Job drawing, mm, ordinate dimensions from the low corner. One solid piece. Round coordinates to 2 decimals unless told otherwise and drop trailing zeros. Write each loop counter-clockwise with the first axis right and the second up, starting at its lowest first coordinate (ties: lowest second). Pieces come first, ordered by that corner, then holes. Notation, with made-up numbers: (-21, -12.75) - (22, -12.75) arc R31 ccw to (22, 26.25) - close; hole circle Ø6 at (46, -2.75). An arc over 180 degrees is marked (long way). Write each question's results on one line, items separated by ' | '.
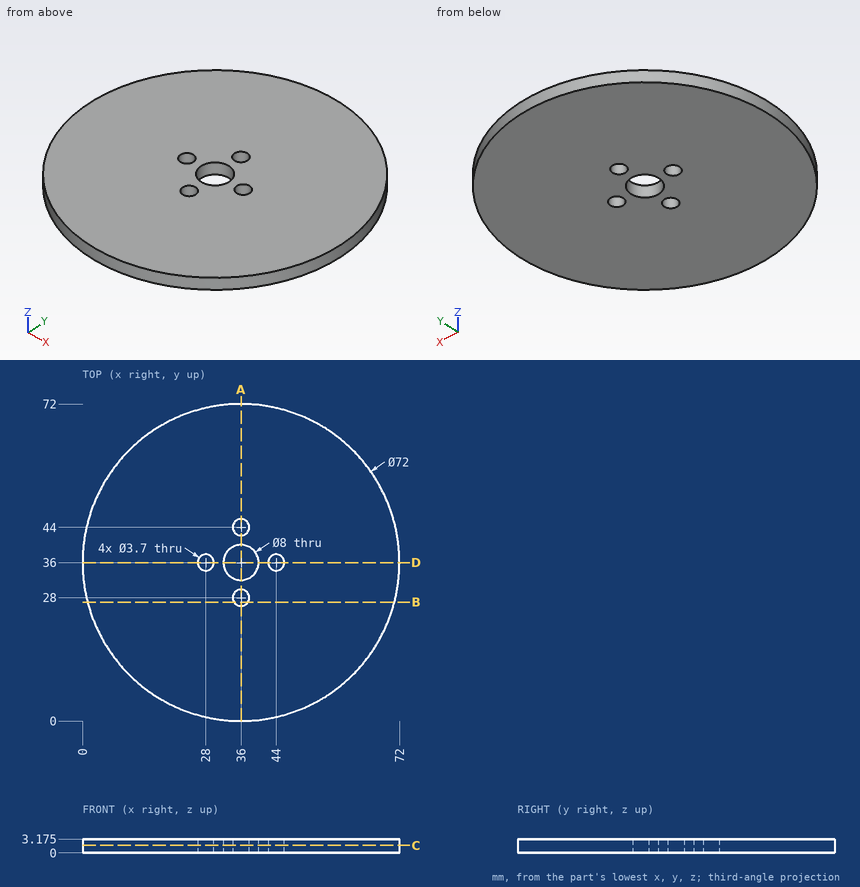
(1) Slice it at C-C, the plane z = 1.7. Write the cut outline in (x, y).
Worked answers:
outline: circle Ø72 at (36, 36); hole circle Ø3.7 at (28, 36); hole circle Ø8 at (36, 36); hole circle Ø3.7 at (36, 28); hole circle Ø3.7 at (36, 44); hole circle Ø3.7 at (44, 36)
(2) Flat gauge pins, fed straight in: pin 1 Ø10.5 at (x, y) = (36, 36) entering from +Z (3 decimals); pin 2 Ø3.5 at (x, y) = (36, 28) entering from -Z; pin 3 Ø1.5 at (y, z) = (41, 2.5) entering from -X. Where does each tip first touch, or does it go through?
Worked answers:
pin 1: stops at z = 3.175 | pin 2: passes through | pin 3: stops at x = 0.25
(3) Drill centre lines: probe 1 along Y at (x, z) = (36, 0.9); probe 2 along Y at (x, z) = (28, 1.9); probe 3 along X at (y, z) = (27.5, 2.05). Where is each one in solid material? Low to high. Write a range as [from, to].
Worked answers:
probe 1: y = [0, 26.15], [29.85, 32], [40, 42.15], [45.85, 72] | probe 2: y = [0.9, 34.15], [37.85, 71.1] | probe 3: x = [1.02, 34.22], [37.78, 70.98]
(4) Slice it at B-B, the plane y = 27. Write the cut outline in (x, z) (3 decimals), and give its area (3 significant figures).
Worked answers:
outline: (1.143, 0) - (34.444, 0) - (34.444, 3.175) - (1.143, 3.175) - close; (37.556, 0) - (70.857, 0) - (70.857, 3.175) - (37.556, 3.175) - close | area: 211 mm2
(5) Slice it at A-A, the plane x = 36. Write the cut outline in (y, z) (3 decimals).
Worked answers:
outline: (0, 0) - (26.15, 0) - (26.15, 3.175) - (0, 3.175) - close; (29.85, 0) - (32, 0) - (32, 3.175) - (29.85, 3.175) - close; (40, 0) - (42.15, 0) - (42.15, 3.175) - (40, 3.175) - close; (45.85, 0) - (72, 0) - (72, 3.175) - (45.85, 3.175) - close
